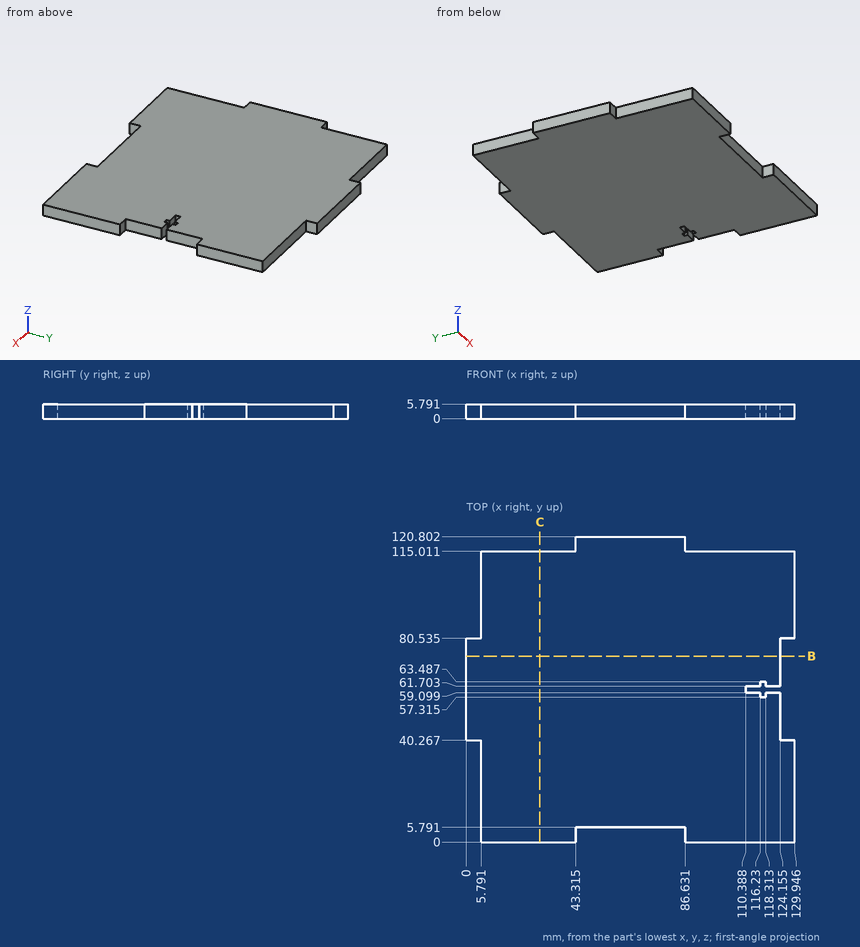
Verification items for this drawing (mm, ordinates from the low corner). Coordinates: 2 decimals unless noted, no trailing zeros. Order: outer loops, then holes, each group sorted by start corner. A loop starts at its lowest first (then second) coordinate and runs counter-clockwise, first axis right, second up. Notation, with made-up numbers: (69, -23) - (75, -23) arc R18 cw to (75, -8) - close; hole circle Ø6 at (-8, 43). An arc over 180 degrees is marked (long way). Answer as a JSON object with one key per item and string values. Group by question number.
Item 1: Sectioned sample at C-C, the plane x = 29. Record the cut outline in (y, z), and give its area (3 significant figures).
Item 2: Depth check by flat-ended pin: pin 1 Ø1.7 at (x, z) = (4, 2.5) entering from -Y; pin 2 Ø1.4 at (y, z) = (62.5, 3) entering from -X; pin 3 Ø1.7 at (y, z) = (118.5, 2) entering from +X; pin 4 Ø3 at (y, z) = (28.5, 2.5) entering from -X. Enter the tip coordinate at first touch or a pass-through.
Item 3: Scan lines: probe 1 along Y at (x, z) = (123, 5.15); probe 2 along X at (y, z) = (37.5, 5.5); probe 3 along X at (y, z) = (55.5, 5.4) (1 decimal). Record each from-to range of solid material in increasing order.
Item 4: Sectioned sample at B-B, the plane y = 73.5. Record the cut outline in (x, z) (1 decimal), and give its area (3 significant figures).
Resolved:
{
 "1": {"outline": "(0, 0) - (115.01, 0) - (115.01, 5.79) - (0, 5.79) - close", "area": "666 mm^2"},
 "2": {"pin 1": "y = 40.27", "pin 2": "x = 0", "pin 3": "x = 86.63", "pin 4": "x = 5.79"},
 "3": {"probe 1": "0 to 59.1, 61.7 to 115.01", "probe 2": "5.79 to 129.95", "probe 3": "0 to 124.2"},
 "4": {"outline": "(0, 0) - (124.2, 0) - (124.2, 5.8) - (0, 5.8) - close", "area": "719 mm^2"}
}
